```python
from build123d import *

# Parameters (mm, degrees)
SKIZZE1_W                                      = 74
SKIZZE1_H                                      = 15
AUFSATZ_LINEAR_AUSTRAGEN1_DEPTH                = 10
SCHNITT_LINEAR_AUSTRAGEN1_REACH                = 61.351
SKIZZE2_W                                      = 71
SKIZZE2_H                                      = 12
FORMSENKUNG_F_R_M3_LINSENSENKSCHRAUB_2_COUNT   = 2
FORMSENKUNG_F_R_M3_LINSENSENKSCHRAUB_2_PITCH   = 34
M3_GEWINDEBOHRUNG1_AT_2_COUNT                  = 2
M3_GEWINDEBOHRUNG1_AT_2_PITCH                  = 65.65
FORMSENKUNG_F_R_M3_LINSENSENKSCHRAUB_3_A_COUNT = 2
FORMSENKUNG_F_R_M3_LINSENSENKSCHRAUB_3_A_PITCH = 65.65


with BuildPart() as part:
    # Skizze1 → Aufsatz-Linear austragen1 (new body)
    with BuildSketch(Plane.XY):
        with Locations((20.392098069, -3.844827586)):
            Rectangle(SKIZZE1_W, SKIZZE1_H)
    extrude(amount=AUFSATZ_LINEAR_AUSTRAGEN1_DEPTH)

    # Skizze2 → Schnitt-Linear austragen1 (cut, up to next)
    with BuildSketch(Plane.XY.offset(10), mode=Mode.PRIVATE) as schnitt_linear_austragen1_sk1:
        with Locations((20.392098069, -3.844827586)):
            Rectangle(SKIZZE2_W, SKIZZE2_H)
    schnitt_linear_austragen1_tool1 = extrude(schnitt_linear_austragen1_sk1.sketch, amount=-SCHNITT_LINEAR_AUSTRAGEN1_REACH, mode=Mode.PRIVATE) & part.part
    add(schnitt_linear_austragen1_tool1.solids().sort_by_distance((20.392098, -3.844828, 10))[0], mode=Mode.SUBTRACT)

    # Skizze10 → Formsenkung f_r M3 Linsensenkschraube mi (revolve, cut)
    with BuildSketch(Plane(origin=(3.392098069, 3.655172414, 5), x_dir=(0, 0, 1), z_dir=(1, 0, 0))):
        Polygon((0, 0), (0, 1.5), (1.7, 1.5), (1.7, 1.45), (3.15, 0), align=None)
    formsenkung_f_r_m3_linsensenkschraube_mi = revolve(axis=Axis((3.392098069, 10.005172414, 5), (0, -1, 0)), mode=Mode.SUBTRACT)

    # Formsenkung f_r M3 Linsensenkschraub 2: Formsenkung f_r M3 Linsensenkschraube mi ×2
    with Locations(*[(i * FORMSENKUNG_F_R_M3_LINSENSENKSCHRAUB_2_PITCH, 0, 0) for i in range(1, FORMSENKUNG_F_R_M3_LINSENSENKSCHRAUB_2_COUNT)]):
        add(formsenkung_f_r_m3_linsensenkschraube_mi, mode=Mode.SUBTRACT)

    # Skizze12 → M3 Gewindebohrung1 (revolve, cut)
    with BuildSketch(Plane(origin=(53.217098069, 3.655172414, 5), x_dir=(0, 0, 1), z_dir=(1, 0, 0))):
        Polygon((0, 0), (0, 1.5), (1.25, 1.5), (1.25, 0.275), (1.525, 0), align=None)
    m3_gewindebohrung1 = revolve(axis=Axis((53.217098069, 10.005172414, 5), (0, -1, 0)), mode=Mode.SUBTRACT)

    # M3 Gewindebohrung1 at 2: M3 Gewindebohrung1 ×2
    with Locations(*[(-i * M3_GEWINDEBOHRUNG1_AT_2_PITCH, 0, 0) for i in range(1, M3_GEWINDEBOHRUNG1_AT_2_COUNT)]):
        add(m3_gewindebohrung1, mode=Mode.SUBTRACT)

    # Skizze13 → Formsenkung f_r M3 Linsensenkschraub 3 (revolve, cut)
    with BuildSketch(Plane(origin=(-12.432901931, -9.844827586, 4.6), x_dir=(0, 0, 1), z_dir=(1, 0, 0))):
        Polygon((0, 0), (0, 1.5), (1.7, 1.5), (1.7, 1.45), (3.15, 0), align=None)
    formsenkung_f_r_m3_linsensenkschraub_3 = revolve(axis=Axis((-12.432901931, -3.494827586, 4.6), (0, -1, 0)), mode=Mode.SUBTRACT)

    # Formsenkung f_r M3 Linsensenkschraub 3 a: Formsenkung f_r M3 Linsensenkschraub 3 ×2
    with Locations(*[(i * FORMSENKUNG_F_R_M3_LINSENSENKSCHRAUB_3_A_PITCH, 0, 0) for i in range(1, FORMSENKUNG_F_R_M3_LINSENSENKSCHRAUB_3_A_COUNT)]):
        add(formsenkung_f_r_m3_linsensenkschraub_3, mode=Mode.SUBTRACT)


solid = part.part
```
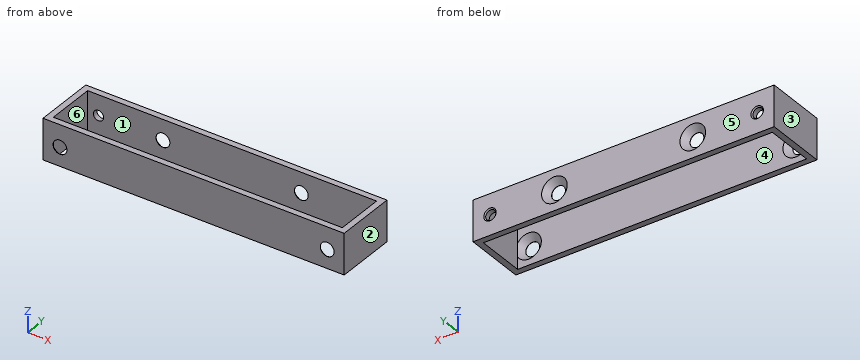
Read the model definition and answer for the solid it produces. Units are mm, in the model's axes. Face numbers are marked on the shaded views. A direction names the side the tool comes from. Round coordinates to 2 decimals unless told otherwise and drop trailing zeros. Loops run counter-clockwise (first coordinate to the right, second up) from the corner with the lowest first, then second, coordinate; pieces in that order, holes last. Notation, with made-up numbers: (67.25, 66) -> (91.25, 66) arc R17 ccw to (91.25, 86) -> close; hole circle Ø4 at (78.25, -18). An arc over 180 degrees is marked (long way). One line per item, written item: value.
1) A cutting plane is placed at B-B (y = -2). Determine the outline of the cut face in (x, z), and give its area (3 significant figures).
Answer list:
outline: (-16.61, 0) -> (-15.11, 0) -> (-15.11, 10) -> (-16.61, 10) -> close; (55.89, 0) -> (57.39, 0) -> (57.39, 10) -> (55.89, 10) -> close
area: 30.0 mm²
2) For the marked faces 1 and 2, determine the directions among +Z, -Z, +X, -X, +Y, -Y from which every point of the face is accessible in a straight line to the end or side of a thin tool.
Answer list:
face 1: +Z, -Z
face 2: +Z, -Z, +X, +Y, -Y
3) A cutting plane is placed at A-A (x = 27). Determine the outline of the cut face in (y, z).
Answer list:
outline: (-11.34, 0) -> (-9.84, 0) -> (-9.84, 10) -> (-11.34, 10) -> close; (2.16, 0) -> (3.66, 0) -> (3.66, 10) -> (2.16, 10) -> close
4) Flat-ended cylindrical pins translate along their axes: P1, Ø2, axis at x = 53.22, z = 5, coming from the -Y side; P2, Ø2, axis at x = 53.22, z = 4.6, coming from the -Y side; P3, Ø2.5, axis at x = 37.39, z = 5, coming from the +Y side. Find the tip coordinate at first contact, or state that the pin passes through.
Answer list:
P1: passes through
P2: stops at y = 2.16
P3: stops at y = -9.84
5) Consider L1, parallel to X at y = -11.3, z = 4.6; L2, parallel to Y at x = 9, z = 5.25; L3, parallel to X at y = -9.75, z = 9. Determine where each line is inside the solid, lowest interval first. Write a range as [from, to].
Answer list:
L1: x = [-16.61, -14.13], [-10.73, 51.52], [54.92, 57.39]
L2: y = [-11.34, -9.84], [2.16, 3.66]
L3: x = [-16.61, -15.11], [55.89, 57.39]
6) The mould has two halves that part along X. Classify the marked faces 3, 4, 5 and 6: pulls with the +X half, pulls with the -X half, needs draft (parallel to the pull), parting line crosses it, or undercut.
Answer list:
face 3: pulls with the -X half
face 4: undercut
face 5: needs draft
face 6: undercut
7) A cutting plane is placed at C-C (z = 4.6). Give the number of separate pieces and of enclosed holes in the cut face, and give its area (3 significant figures).
Answer list:
separate pieces: 6
enclosed holes: 0
area: 222 mm²
